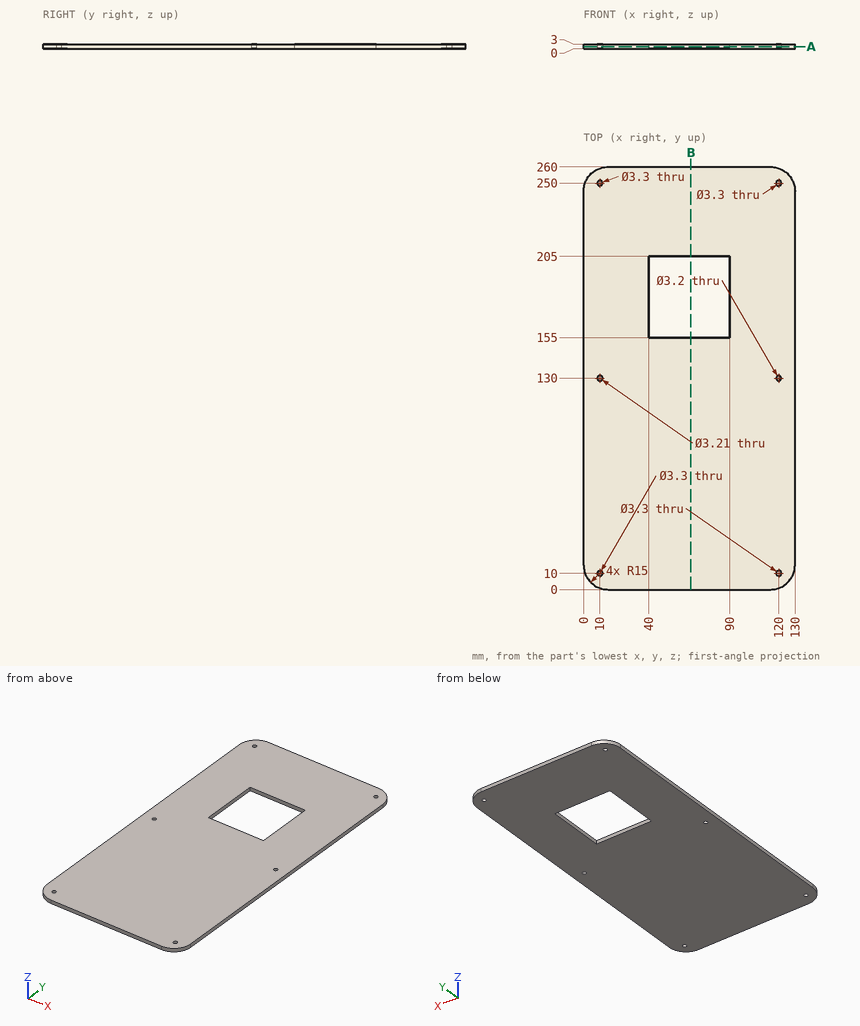
Could you check a few things on this drawing? It's one solid part, dimensions in mm from its lowest x, y, z. Give positions to 0.01 mm unless a question says otherwise; leave off trailing zeros. Order: outer loops, then holes, each group sorted by start corner. A loop starts at its lowest first (then second) coordinate and runs counter-clockwise, first axis right, second up. Notation, with made-up numbers: (3.5, 27) -> (19.5, 27) arc R18 cw to (19.5, 32) -> close; hole circle Ø11 at (46.5, 2). An arc over 180 degrees is marked (long way). Answer in a Markdown table with one row per item. Add a question column.
Item 1: Imagine slicing it at A-A (z = 1.4). List the corners of the cut face in (x, y) for me (3 decimals).
Item 2: Please list where these lines run through material, in increasing order: probe 1 along X at (y, z) = (130, 2.2) (3 decimals); probe 2 along Y at (x, z) = (60, 2.8); probe 3 along X at (y, z) = (182, 1.05).
Item 3: I'm going to push a flat-ended pin straight in: P1, Ø5, axis at x = 10, y = 130, coming from the +Z side. Where does the tip first touch, or does it pass through?
Item 4: Imagine slicing it at B-B (x = 66). List the corners of the cut face in (y, z) for me, and give its area (3 significant figures).
Result:
| question | item | result |
|---|---|---|
| 1 | outline | (0, 15) arc R15 ccw to (15, 0) -> (115, 0) arc R15 ccw to (130, 15) -> (130, 245) arc R15 ccw to (115, 260) -> (15, 260) arc R15 ccw to (0, 245) -> close; hole circle Ø3.3 at (10, 10); hole circle Ø3.3 at (10, 250); hole circle Ø3.21 at (10, 130); hole (40, 155) -> (90, 155) -> (90, 205) -> (40, 205) -> close; hole circle Ø3.3 at (120, 10); hole circle Ø3.3 at (120, 250); hole circle Ø3.2 at (120, 130) |
| 2 | probe 1 | 0 to 8.395, 11.605 to 118.4, 121.6 to 130 |
| 2 | probe 2 | 0 to 155, 205 to 260 |
| 2 | probe 3 | 0 to 40, 90 to 130 |
| 3 | P1 | z = 3 |
| 4 | outline | (0, 0) -> (155, 0) -> (155, 3) -> (0, 3) -> close; (205, 0) -> (260, 0) -> (260, 3) -> (205, 3) -> close |
| 4 | area | 630 mm2 |
